For this review, use the dimensioned drawing (mm, ordinates from the lowest corner) and the shaded views. Coordinates: 2 decimals unless noted, no trailing zeros. Loops run counter-clockwise (first coordinate to the right, second up) from the corner with the lowest first, then second, coordinate; pieces in that order, holes last. Notation, with made-up numbers: (51, 29.25) -> (102, 29.25) arc R30 cw to (102, 66.25) -> close; hole circle Ø5 at (83.25, 40.5). An arc over 180 degrees is marked (long way). One line per question, with ' | ' between items. Start each with the question number.
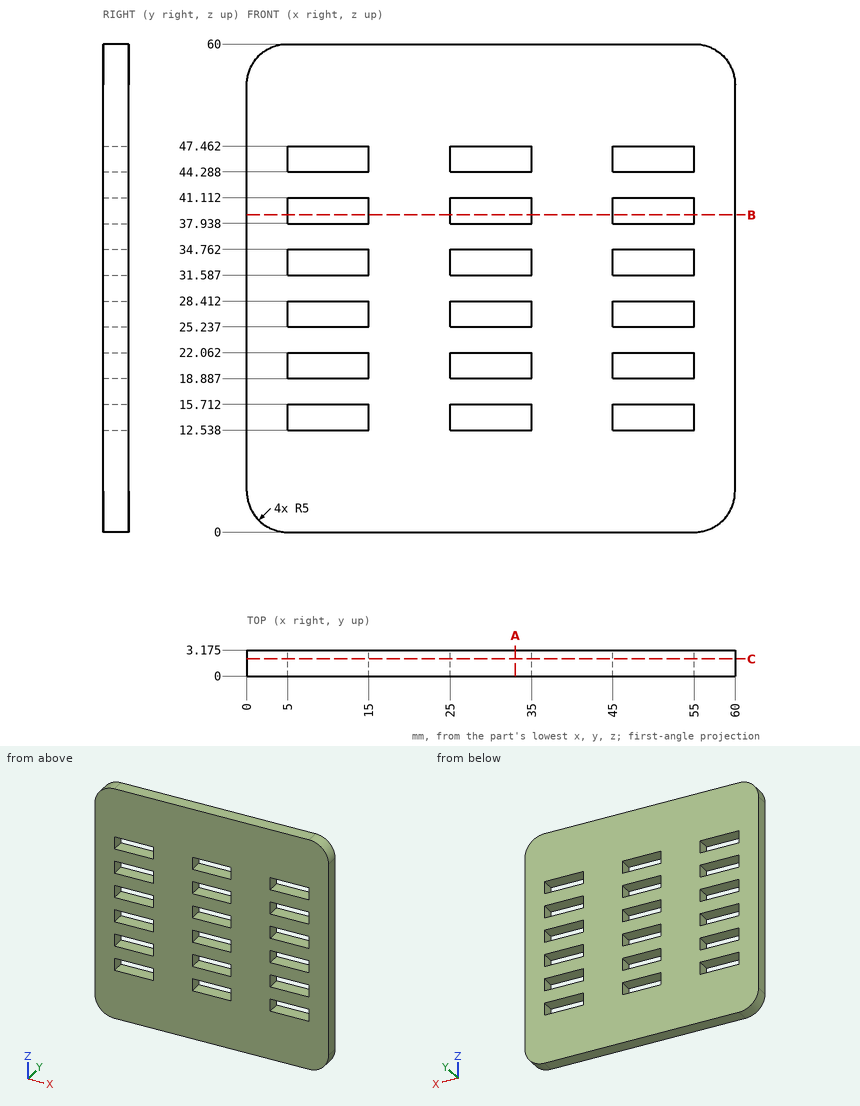
1) Consider section C-C, the plane y = 2.1. Give the number of separate pieces and of enclosed holes in the cut face, plus the area to 3 significant figures.
2) Consider section A-A, the plane x = 33. Write out the cut boundary in (y, z) (1 decimal).
3) Wall thickness on L1, parallel to X at y = 0.35, z = 45; L2, parallel to X at y = 0.7, z = 3.5; L3, parallel to X at y = 2.1, z = 3: over which ranges is each line inside the solid? List them lowest first.
4) Consider section B-B, the plane z = 39. Write out the cut boundary in (x, y) (1 decimal).
Filled sheet:
1) separate pieces: 1 | enclosed holes: 18 | area: 3,010 mm^2
2) outline: (0, 0) -> (3.2, 0) -> (3.2, 12.5) -> (0, 12.5) -> close; (0, 15.7) -> (3.2, 15.7) -> (3.2, 18.9) -> (0, 18.9) -> close; (0, 22.1) -> (3.2, 22.1) -> (3.2, 25.2) -> (0, 25.2) -> close; (0, 28.4) -> (3.2, 28.4) -> (3.2, 31.6) -> (0, 31.6) -> close; (0, 34.8) -> (3.2, 34.8) -> (3.2, 37.9) -> (0, 37.9) -> close; (0, 41.1) -> (3.2, 41.1) -> (3.2, 44.3) -> (0, 44.3) -> close; (0, 47.5) -> (3.2, 47.5) -> (3.2, 60) -> (0, 60) -> close
3) L1: 0 to 5, 15 to 25, 35 to 45, 55 to 60 | L2: 0.23 to 59.77 | L3: 0.42 to 59.58
4) outline: (0, 0) -> (5, 0) -> (5, 3.2) -> (0, 3.2) -> close; (15, 0) -> (25, 0) -> (25, 3.2) -> (15, 3.2) -> close; (35, 0) -> (45, 0) -> (45, 3.2) -> (35, 3.2) -> close; (55, 0) -> (60, 0) -> (60, 3.2) -> (55, 3.2) -> close
